Part model, mm, in its own coordinate system. A direction names the side the tool comes from. Give positions to 0.01 mm unless a question says otherwise; leave off trailing zeros. Write each loop counter-clockwise with the first axis right and the second up, starting at its lowest first coordinate (ties: lowest second). Pieces come first, ordered by that corner, then holes. Notation, with made-up numbers: (82.5, 76.5) - (105.5, 76.5) arc R30 ccw to (105.5, 114.5) - close; hole circle Ø7 at (1, -40). An arc over 180 degrees is marked (long way). Answer in a Markdown table with one row per item. Add a question column.
1. Probe line 1 along Z through (x, y) = (15, 8.25); line 2 along X through (y, z) = (4.75, -10.5); line 3 along Y through (x, z) = (-6.5, -11.25). List the from-to ranges inside material, lowest first.
2. Band-saw the part on B-B on z = -9. Write the cut outline in (x, y).
3. Band-saw the part on C-C on x = -9.5. Write the cut outline in (y, z).
4. Which spindle directions (+Z, -Z, +X, -X, +Y, -Y) get a long thin tool onto all of the face, cutting with end or side? Do faces 1 (the flat face through (-27.852, 12, -6)), 2 (the flat face through (19.148, 12, -7)). Say none if no direction does.
5. Drop a flat-ended pin along its axis: pin 1 Ø7.5 at (x, z) = (-15.5, -13) entering from -Y. Give the stop position or say it passes through.
6. Band-saw the part on A-A on y = 7.75. Write the cut outline in (x, z), plus the area to 3 significant figures.
7. Pull direction X, two halves, no side cores. Call faces 3 (the cylindrical face through (-3.53, 24.199, -19.866)), 4 (the cylindrical face through (-27.567, 11.914, -19.85)), 5 (the flat face through (-26.852, 12, -7)): released by +X, released by -X, zero draft, split by the parting line, or undercut.
```python
from build123d import *

# Parameters (mm, degrees)
SKETCH_1_W          = 48
SKETCH_1_H          = 27
EXTRUDE_1_DEPTH     = 24.5
FILLET_1_R          = 1
SKETCH_4_W          = 46
SKETCH_4_H          = 25
CUT_EXTRUDE_1_DEPTH = 23.5


with BuildPart() as part:
    # ｽｹｯﾁ1 → ﾎﾞｽ - 押し出し1 (new body)
    with BuildSketch(Plane(origin=(0, 0, 0), x_dir=(1, 0, 0), z_dir=(0, 1, 0))):
        with Locations((-3.851977642, 6.650666667)):
            Rectangle(SKETCH_1_W, SKETCH_1_H)
    extrude(amount=EXTRUDE_1_DEPTH)

    # ﾌｨﾚｯﾄ1
    fillet_1_edges = [part.edges().sort_by_distance(p)[0] for p in [
        (20.148022358, 24.5, -6.650666667),
        (-3.851977642, 24.5, -20.150666667),
        (-27.851977642, 24.5, -6.650666667),
        (-3.851977642, 24.5, 6.849333333),
        (-27.851977642, 12.25, -20.150666667),
        (20.148022358, 12.25, -20.150666667),
        (20.148022358, 12.25, 6.849333333),
        (-27.851977642, 12.25, 6.849333333),
    ]]
    fillet(fillet_1_edges, radius=FILLET_1_R)

    # ｽｹｯﾁ4 → ｶｯﾄ - 押し出し1 (cut)
    with BuildSketch(Plane.XZ):
        with Locations((-3.851977642, -6.650666667)):
            Rectangle(SKETCH_4_W, SKETCH_4_H)
    extrude(amount=-CUT_EXTRUDE_1_DEPTH, mode=Mode.SUBTRACT)


solid = part.part
```
Values:
| question | item | result |
|---|---|---|
| 1 | line 1 | z = -20.15 to -19.15, 5.85 to 6.85 |
| 1 | line 2 | x = -27.85 to -26.85, 19.15 to 20.15 |
| 1 | line 3 | y = 23.5 to 24.5 |
| 2 | outline | (-27.85, 0) - (-26.85, 0) - (-26.85, 23.5) - (19.15, 23.5) - (19.15, 0) - (20.15, 0) - (20.15, 23.5) arc R1 ccw to (19.15, 24.5) - (-26.85, 24.5) arc R1 ccw to (-27.85, 23.5) - close |
| 3 | outline | (0, -20.15) - (23.5, -20.15) arc R1 ccw to (24.5, -19.15) - (24.5, 5.85) arc R1 ccw to (23.5, 6.85) - (0, 6.85) - (0, 5.85) - (23.5, 5.85) - (23.5, -19.15) - (0, -19.15) - close |
| 4 | face 1 | +Z, -Z, -X, +Y, -Y |
| 4 | face 2 | -Y |
| 5 | pin 1 | stops at y = 23.5 |
| 6 | outline | (-27.85, -19.15) arc R1 ccw to (-26.85, -20.15) - (19.15, -20.15) arc R1 ccw to (20.15, -19.15) - (20.15, 5.85) arc R1 ccw to (19.15, 6.85) - (-26.85, 6.85) arc R1 ccw to (-27.85, 5.85) - close; hole (-26.85, -19.15) - (19.15, -19.15) - (19.15, 5.85) - (-26.85, 5.85) - close |
| 6 | area | 145 mm² |
| 7 | face 3 | zero draft |
| 7 | face 4 | released by -X |
| 7 | face 5 | undercut |
